Part model, mm, in its own coordinate system. A direction names the side the tool comes from. Give positions to 0.01 mm unless a question says otherwise; leave off trailing zeros. Loops run counter-clockwise (first coordinate to the right, second up) from the corner with the lowest first, then second, coordinate; pieces in that order, holes last. Notation, with made-up numbers: (70.5, 27.25) -> (128.5, 27.25) arc R26 ccw to (128.5, 48.25) -> close; hole circle Ø10 at (73.25, -8). An arc over 180 degrees is marked (long way). Write item = value, one per line.
from build123d import *
from build123d.topology import SkipClean

# Parameters (mm, degrees)
SALIENTE_EXTRUIR2_DEPTH      = 20
SALIENTE_EXTRUIR3_START      = -2.463797
SALIENTE_EXTRUIR3_DEPTH      = 2.463797
SALIENTE_EXTRUIR4_DEPTH      = 2.463797195
CROQUIS4_R                   = 2
CROQUIS4_R_2                 = 3.5
SALIENTE_EXTRUIR5_DEPTH      = 10
CORTAR_EXTRUIR1_DEPTH        = 10
CORTAR_EXTRUIR1_DEPTH_BACK   = 19
CROQUIS5_W                   = 10.904508264
CROQUIS5_H                   = 15.264086628
SALIENTE_EXTRUIR6_DEPTH      = 9.255106
SALIENTE_EXTRUIR6_DEPTH_BACK = 10.025
CROQUIS7_W                   = 23.956346688
CROQUIS7_H                   = 15.277003438
CORTAR_EXTRUIR2_DEPTH        = 103.636657602
CROQUIS9_W                   = 4
CROQUIS9_H                   = 12.8
CORTAR_EXTRUIR3_DEPTH        = 44.32026299
SALIENTE_EXTRUIR14_DEPTH     = 17.727594
CROQUIS11_R                  = 1.7
SALIENTE_EXTRUIR15_DEPTH     = 2
SALIENTE_EXTRUIR16_DEPTH     = 12.8


with BuildPart() as part:
    # Croquis1 → Saliente-Extruir2 (new body)
    with BuildSketch(Plane.XY):
        Polygon((60.885724234, -9.113797195), (97.885724234, -9.113797195), (97.885724234, 8.613797195), (60.885724234, 8.613797195), (60.885724234, 6.15), (94.885724234, 6.15), (94.885724234, -6.65), (60.885724234, -6.65), align=None)
    extrude(amount=SALIENTE_EXTRUIR2_DEPTH)

    # Croquis2 → Saliente-Extruir3 (add)
    with SkipClean():  # the faces are left unmerged after this step: merging them gives an invalid solid
        with BuildSketch(Plane(origin=(0, 8.613797195, 0), x_dir=(1, 0, 0), z_dir=(0, 1, 0)).offset(SALIENTE_EXTRUIR3_START)):
            with BuildLine():
                ThreePointArc((71.814275766, 2), (70.308416296, 0.672909982), (68.417392018, 0))
                Line((68.417392018, 0), (97.885724234, 0))
                Line((97.885724234, 0), (71.814275766, 9.255105503))
                Line((71.814275766, 9.255105503), (71.814275766, 2))
            make_face()
            Polygon((50.000330077, 0), (60.885724234, -8.516201314), (60.885724234, 0), align=None)
        extrude(amount=SALIENTE_EXTRUIR3_DEPTH)

    # Croquis3 → Saliente-Extruir4 (add)
    with SkipClean():  # the faces are left unmerged after this step: merging them gives an invalid solid
        with BuildSketch(Plane.XZ.offset(9.113797195)):
            Polygon((60.885724234, 0), (60.885724234, 8.516201314), (50.000330077, 0), align=None)
            with BuildLine():
                Line((94.885724234, 0), (68.417392018, 0))
                ThreePointArc((68.417392018, 0), (70.308416296, -0.672909982), (71.814275766, -2))
                Line((71.814275766, -2), (71.814275766, -9.255105503))
                Line((71.814275766, -9.255105503), (97.885724234, 0))
                Line((97.885724234, 0), (94.885724234, 0))
            make_face()
        extrude(amount=-SALIENTE_EXTRUIR4_DEPTH)

    # Croquis4 → Saliente-Extruir5 (add)
    # profile 1 of 4: a face of its own
    with SkipClean():  # the faces are left unmerged after this step: merging them gives an invalid solid
        with BuildSketch(Plane(origin=(0, 0, 0), x_dir=(-1, 0, 0), z_dir=(0, 0, -1))):
            with BuildLine():
                ThreePointArc((-84.385724234, 12.113797195), (-81.296227313, 10.065720048), (-77.885724234, 8.613797195))
                Line((-77.885724234, 8.613797195), (-97.885724234, 8.613797195))
                ThreePointArc((-97.885724234, 8.613797195), (-94.475221154, 10.065720048), (-91.385724234, 12.113797195))
                ThreePointArc((-91.385724234, 12.113797195), (-87.885724234, 15.613797195), (-84.385724234, 12.113797195))
            make_face()
            with Locations((-87.885724234, 12.113797195)):
                Circle(CROQUIS4_R, mode=Mode.SUBTRACT)
        # profile 2 of 4: a face of its own
        with BuildSketch(Plane(origin=(0, 0, 0), x_dir=(-1, 0, 0), z_dir=(0, 0, -1))):
            with BuildLine():
                ThreePointArc((-91.385724234, -12.613797195), (-90.360597982, -10.138923475), (-87.885724275, -9.113797195))
                Line((-87.885724275, -9.113797195), (-97.885724234, -9.113797195))
                ThreePointArc((-97.885724234, -9.113797195), (-94.475221154, -10.565720048), (-91.385724234, -12.613797195))
            make_face()
        # profile 3 of 4: a face of its own
        with BuildSketch(Plane(origin=(0, 0, 0), x_dir=(-1, 0, 0), z_dir=(0, 0, -1))):
            with BuildLine():
                ThreePointArc((-84.385724234, -12.613797195), (-81.296227313, -10.565720048), (-77.885724234, -9.113797195))
                Line((-77.885724234, -9.113797195), (-87.885724275, -9.113797195))
                ThreePointArc((-87.885724275, -9.113797195), (-85.410850514, -10.138923446), (-84.385724234, -12.613797195))
            make_face()
        # profile 4 of 4: a face of its own
        with BuildSketch(Plane(origin=(0, 0, 0), x_dir=(-1, 0, 0), z_dir=(0, 0, -1))):
            with Locations((-87.885724234, -12.613797195)):
                Circle(CROQUIS4_R_2)
            with Locations((-87.885724234, -12.613797195)):
                Circle(CROQUIS4_R, mode=Mode.SUBTRACT)
        extrude(amount=-SALIENTE_EXTRUIR5_DEPTH)

    # Croquis5 → Cortar-Extruir1 (cut, two sides: drawn at the far end of the back side and taken through both)
    with SkipClean():  # the faces are left unmerged after this step: merging them gives an invalid solid
        with BuildSketch(Plane(origin=(0, 0, 0), x_dir=(-1, 0, 0), z_dir=(0, 0, -1)).offset(-CORTAR_EXTRUIR1_DEPTH_BACK)):
            with Locations((-89.39295043, -0.250144717)):
                Rectangle(CROQUIS5_W, CROQUIS5_H)
        extrude(amount=CORTAR_EXTRUIR1_DEPTH + CORTAR_EXTRUIR1_DEPTH_BACK, mode=Mode.SUBTRACT)

    # Croquis7 → Saliente-Extruir6 (add, two sides: drawn at the far end of the back side and taken through both)
    with SkipClean():  # the faces are left unmerged after this step: merging them gives an invalid solid
        with BuildSketch(Plane(origin=(0, 0, 0), x_dir=(-1, 0, 0), z_dir=(0, 0, -1)).offset(-SALIENTE_EXTRUIR6_DEPTH_BACK)):
            with Locations((-72.90755089, -0.256603122)):
                Rectangle(CROQUIS7_W, CROQUIS7_H)
        extrude(amount=SALIENTE_EXTRUIR6_DEPTH + SALIENTE_EXTRUIR6_DEPTH_BACK)

    # Croquis8 → Cortar-Extruir2 (cut, through all)
    with SkipClean():  # the faces are left unmerged after this step: merging them gives an invalid solid
        with BuildSketch(Plane.XZ.offset(7.895104841)):
            with BuildLine():
                ThreePointArc((71.814275766, -2), (70.308416296, -0.672909982), (68.417392018, 0))
                Line((68.417392018, 0), (60.929377546, 0))
                Line((60.929377546, 0), (60.929377546, -9.255105503))
                Line((60.929377546, -9.255105503), (71.814275766, -9.255105503))
                Line((71.814275766, -9.255105503), (71.814275766, -2))
            make_face()
            Polygon((84.885724234, -4.614871003), (71.814275766, -9.255105503), (84.885724234, -9.255105503), align=None)
        extrude(amount=-CORTAR_EXTRUIR2_DEPTH, mode=Mode.SUBTRACT)


with BuildPart() as cortar_extruir2_kept_piece:
    # of the separate pieces the step leaves, the one the design keeps (cortar_extruir2_pieces_kept)
    add(part.part.solids().sort_by_distance((60.885724234, -9.113797195, 0))[0])

    # Croquis9 → Cortar-Extruir3 (cut, through all)
    with BuildSketch(Plane(origin=(84.885724234, 0, 0), x_dir=(0, 0, -1), z_dir=(1, 0, 0))):
        with Locations((-2, -0.25)):
            Rectangle(CROQUIS9_W, CROQUIS9_H)
    extrude(amount=-CORTAR_EXTRUIR3_DEPTH, mode=Mode.SUBTRACT)

    # Croquis10 → Saliente-Extruir14 (add)
    with SkipClean():  # the faces are left unmerged after this step: merging them gives an invalid solid
        with BuildSketch(Plane.XZ.offset(9.113797195)):
            Polygon((71.814275766, -9.255105503), (71.814275766, -10.980236396), (97.885724234, -2), (97.885724234, 0), (97.885724234, 0.393932893), (71.814275766, -8.86117261), align=None)
        extrude(amount=-SALIENTE_EXTRUIR14_DEPTH)

    # Croquis11 → Saliente-Extruir15 (add)
    # profile 1 of 2: a face of its own
    with SkipClean():  # the faces are left unmerged after this step: merging them gives an invalid solid
        with BuildSketch(Plane(origin=(0, 0, 0), x_dir=(-1, 0, 0), z_dir=(0, 0, -1))):
            with BuildLine():
                Line((-68.417392018, -9.113797195), (-50.000330077, -9.113797195))
                Line((-50.000330077, -9.113797195), (-50.000330077, -17.113797195))
                ThreePointArc((-50.000330077, -17.113797195), (-50.586116515, -18.528010757), (-52.000330077, -19.113797195))
                Line((-52.000330077, -19.113797195), (-66.417392018, -19.113797195))
                ThreePointArc((-66.417392018, -19.113797195), (-67.831605581, -18.528010757), (-68.417392018, -17.113797195))
                Line((-68.417392018, -17.113797195), (-68.417392018, -9.113797195))
            make_face()
            with Locations(Location((-65.166367035, -13.113797195, 0), (0, 0, 180))):
                Circle(CROQUIS11_R, mode=Mode.SUBTRACT)
            with Locations(Location((-53.166367035, -13.113797195, 0), (0, 0, 180))):
                Circle(CROQUIS11_R, mode=Mode.SUBTRACT)
        # profile 2 of 2: a face of its own
        with BuildSketch(Plane(origin=(0, 0, 0), x_dir=(-1, 0, 0), z_dir=(0, 0, -1))):
            with BuildLine():
                Line((-50.000330077, 8.613797195), (-68.814275766, 8.613797195))
                Line((-68.814275766, 8.613797195), (-68.814275766, 16.613797195))
                ThreePointArc((-68.814275766, 16.613797195), (-68.228489329, 18.028010757), (-66.814275766, 18.613797195))
                Line((-66.814275766, 18.613797195), (-52.000330077, 18.613797195))
                ThreePointArc((-52.000330077, 18.613797195), (-50.586116515, 18.028010757), (-50.000330077, 16.613797195))
                Line((-50.000330077, 16.613797195), (-50.000330077, 8.613797195))
            make_face()
            with Locations((-53.166367035, 12.613797195)):
                Circle(CROQUIS11_R, mode=Mode.SUBTRACT)
            with Locations((-65.166367035, 12.613797195)):
                Circle(CROQUIS11_R, mode=Mode.SUBTRACT)
        extrude(amount=-SALIENTE_EXTRUIR15_DEPTH)

    # Croquis12 → Saliente-Extruir16 (add)
    with SkipClean():  # the faces are left unmerged after this step: merging them gives an invalid solid
        with BuildSketch(Plane(origin=(0, -6.65, 0), x_dir=(1, 0, 0), z_dir=(0, 1, 0))):
            Polygon((60.885724234, -8.516201314), (52.556726704, -2), (55.113123331, -2), (60.885724234, -6.516201314), align=None)
        extrude(amount=SALIENTE_EXTRUIR16_DEPTH)


solid = cortar_extruir2_kept_piece.part
1) Pull direction Z, two halves, no side cores. Call faces 4 (the face through (59, -14, 2)), 5 (the face through (89, -7.882, 8)), 6 (the face through (84.667, -0.374, -6.553)), 7 (the face through (51, -9.114, 1)): pulls with the +Z half, pulls with the -Z half, needs draft (parallel to the pull), parting line crosses it, or undercut.
Resolved:
face_4 = pulls with the +Z half
face_5 = undercut
face_6 = pulls with the -Z half
face_7 = needs draft
2) Slice it at A-A, the plane y = -4. List the corners of the cut face in (x, z) (3 decimals), and give its area (3 significant figures).
Resolved:
outline = (52.557, 2) -> (55.113, 2) -> (60.886, 6.516) -> (60.886, 8.516) -> close; (60.929, 4) -> (84.886, 4) -> (84.886, 10.025) -> (60.929, 10.025) -> close; (68.417, 0) arc R5.307 cw to (71.814, -2) -> (71.814, -10.98) -> (97.886, -2) -> (97.886, 20) -> (94.886, 20) -> (94.886, 0) -> (96.776, 0) -> (84.886, -4.221) -> (84.886, 0) -> close
area = 365 mm²
3) Slice it at D-D, the plane z = 5.5. List the corners of the cut face in (x, y), and give its area (3 significant figures).
Resolved:
outline = (57.03, -9.11) -> (77.89, -9.11) arc R20.29 cw to (84.39, -12.61) arc R3.5 ccw to (91.39, -12.61) arc R20.29 cw to (97.89, -9.11) -> (97.89, 8.61) arc R20.29 cw to (91.39, 12.11) arc R3.5 ccw to (84.39, 12.11) arc R20.29 cw to (77.89, 8.61) -> (57.03, 8.61) -> close; hole (59.59, -6.65) -> (60.93, -6.65) -> (60.93, 6.15) -> (59.59, 6.15) -> close; hole (84.89, -7.88) -> (94.85, -7.88) -> (94.85, -6.65) -> (94.89, -6.65) -> (94.89, 6.15) -> (94.85, 6.15) -> (94.85, 7.38) -> (84.89, 7.38) -> close; hole circle Ø4 at (87.89, -12.61); hole circle Ø4 at (87.89, 12.11)
area = 656 mm²
4) Slice it at C-C, the plane x = 54. List the corners of the cut face in (y, z).
Resolved:
outline = (-19.11, 0) -> (-14.6, 0) -> (-14.6, 2) -> (-19.11, 2) -> close; (-11.63, 0) -> (-6.65, 0) -> (-6.65, 2) -> (6.15, 2) -> (6.15, 0) -> (11.13, 0) -> (11.13, 2) -> (8.61, 2) -> (8.61, 3.13) -> (-9.11, 3.13) -> (-9.11, 2) -> (-11.63, 2) -> close; (14.1, 0) -> (18.61, 0) -> (18.61, 2) -> (14.1, 2) -> close
5) Which spindle directions (+Z, -Z, +X, -X, +Y, -Y) get a long thin tool onto all of the face, cutting with end or side? Do faces 1 (the face through (71.814, 0, -7)), 2 (the face through (83.941, -7, 15)), 3 (the face through (87.963, -16.113, 4.93)). Say none if no direction does.
Resolved:
face_1 = -Z, -X, +Y, -Y
face_2 = none
face_3 = +Z, -Z, -Y
6) Drill centre lines: line 1 along Y through (x, z) = (72.5, 12.5); line 2 along X through (y, z) = (6.5, 18.5); line 3 along Y through (x, z) = (92.5, 18). Where is each one in solid material? Low to high. Write a range as [from, to].
Resolved:
line_1 = [-9.11, -6.65], [6.15, 8.61]
line_2 = [60.89, 83.94], [94.85, 97.89]
line_3 = [-9.11, -7.88], [7.38, 8.61]
7) Slice it at B-B, the plane z = 18. List the corners of the cut face in (x, y), and give its area (3 significant figures).
Resolved:
outline = (60.89, -9.11) -> (97.89, -9.11) -> (97.89, 8.61) -> (60.89, 8.61) -> (60.89, 6.15) -> (83.94, 6.15) -> (83.94, 7.38) -> (94.85, 7.38) -> (94.85, 6.15) -> (94.89, 6.15) -> (94.89, -6.65) -> (94.85, -6.65) -> (94.85, -7.88) -> (83.94, -7.88) -> (83.94, -6.65) -> (60.89, -6.65) -> close
area = 194 mm²
8) Drop flat-ended pins along their axis: P1, Ø3, axis at x = 76, z = 4.5, coming from the -Y side; P2, Ø0.6, axis at y = -12.5, z = 1.5, coming from the +X side; P3, Ø5.5, axis at x = 53.17, y = -13.11, coming from the -Z side; P4, Ø2, axis at x = 51.5, z = 0.5, coming from the -Y side. Give the stop position or say it passes through.
Resolved:
P1 = -9.11
P2 = 91.92
P3 = 0
P4 = -19.11
